```python
from build123d import *

# Parameters (mm, degrees)
F0_R     = 2.5
F1_DEPTH = 4
F2_R     = 2
F3_R     = 1
F4_R     = 0.7
F5_R     = 0.2
F6_R     = 2
F7_R     = 5


with BuildPart() as f1:
    # F0 (on Top) → F1 (new body)
    with BuildSketch(Plane.XY):
        with BuildLine():
            Line((-44, 8.8584928558), (-44, 4.8989794856))
            ThreePointArc((-44, 4.8989794856), (-49.974680765, 0.50254481), (-45, -5))
            Line((-45, -5), (-45, -6.2))
            Line((-45, -6.2), (0, -6.2))
            Line((0, -6.2), (0, -5))
            ThreePointArc((0, -5), (4.974680765, 0.50254481), (-1, 4.8989794856))
            Line((-1, 4.8989794856), (-1, 8.8584928558))
            ThreePointArc((-1, 8.8584928558), (2.3623310777, 10.7048643976), (3.7, 14.3))
            Line((3.7, 14.3), (3.7, 30.6369656558))
            ThreePointArc((3.7, 30.6369656558), (4.7588909504, 35.5339351103), (1.0395584541, 38.8907380037))
            Line((1.0395584541, 38.8907380037), (-4.1791089332, 40))
            Line((-4.1791089332, 40), (-40.8208910668, 40))
            Line((-40.8208910668, 40), (-46.0395584541, 38.8907380037))
            ThreePointArc((-46.0395584541, 38.8907380037), (-49.7588909504, 35.5339351103), (-48.7, 30.6369656558))
            Line((-48.7, 30.6369656558), (-48.7, 14.3))
            ThreePointArc((-48.7, 14.3), (-47.3623310777, 10.7048643976), (-44, 8.8584928558))
        make_face()
        with Locations((-45, 0)):
            Circle(F0_R, mode=Mode.SUBTRACT)
        Circle(F0_R, mode=Mode.SUBTRACT)
        with Locations((-45, 34)):
            Circle(F0_R, mode=Mode.SUBTRACT)
        with Locations((0, 34)):
            Circle(F0_R, mode=Mode.SUBTRACT)
    extrude(amount=F1_DEPTH)

    # F2
    f2_edges = [f1.edges().sort_by_distance(p)[0] for p in [
        (-44, 8.858493, 2),
        (-1, 8.858493, 2),
    ]]
    fillet(f2_edges, radius=F2_R)

    # F3
    f3_edges = [f1.edges().sort_by_distance(p)[0] for p in [
        (-1, 4.898979, 2),
        (-44, 4.898979, 2),
    ]]
    fillet(f3_edges, radius=F3_R)

    # F4
    f4_edges = [f1.edges().sort_by_distance(p)[0] for p in [
        (-45, -5, 2),
        (0, -5, 2),
    ]]
    fillet(f4_edges, radius=F4_R)

    # F5
    f5_edges = [f1.edges().sort_by_distance(p)[0] for p in [
        (-45, -6.2, 2),
        (0, -6.2, 2),
    ]]
    fillet(f5_edges, radius=F5_R)

    # F6
    f6_edges = [f1.edges().sort_by_distance(p)[0] for p in [
        (-48.7, 30.636966, 2),
        (3.7, 30.636966, 2),
    ]]
    fillet(f6_edges, radius=F6_R)

    # F7
    f7_edges = [f1.edges().sort_by_distance(p)[0] for p in [
        (-40.820891, 40, 2),
        (-4.179109, 40, 2),
    ]]
    fillet(f7_edges, radius=F7_R)


solid = f1.part
```
For this review, take the finished solid that the model builds, in its own axes (mm). A direction names the side the tool comes from. Round coordinates to 2 decimals unless told otherwise and drop trailing zeros. Loops run counter-clockwise (first coordinate to the right, second up) from the corner with the lowest first, then second, coordinate; pieces in that order, holes last.
Q1. Insertion check: pin 1 Ø2 at (y, z) = (11.5, 3) entering from -X; pin 2 Ø4 at (x, y) = (-45, 34) entering from +Z; pin 3 Ø1.2 at (y, z) = (22.5, 2.5) entering from +X; pin 4 Ø1.1 at (y, z) = (6.5, 2.5) entering from -X. Each pin has a flat end and moves straight along its axis. Give the tip position at first contact, or say it passes through.
Result sheet:
pin 1: stops at x = -48.4
pin 2: passes through
pin 3: stops at x = 3.7
pin 4: stops at x = -44
Q2. Add section B-B on z = 0.8. Give the number of separate pieces and of enclosed holes in the cut face, plus the area to 3 significant figures.
Result sheet:
separate pieces: 1
enclosed holes: 4
area: 2,290 mm2
Q3. Machinability: for faces 1 (the face through (-47.783, 11.259, 1.972)), 2 (the face through (2.73, 11.18, 1.97)), 3 (the face through (-23, 17, 0)), which of the approach directions +Z, -Z, +X, -X, +Y, -Y give a long, thin tool a straight path to every point of the face, cutting with its end or side? Answer none if there is none.
Result sheet:
face 1: +Z, -Z, -X
face 2: +Z, -Z, +X
face 3: -Z, +X, -X, +Y, -Y
Q4. Mouldability with a two-part tool opening along X and no side actions: class faces 4 (the face through (-23, -6.2, 2)), 5 (the face through (-1.28, 39.384, 1.972)), 6 (the face through (-42.69, -0.96, 1.97)) as +X half, -X half, draft (parallel to the pull), parting line (faces both ways), or undercut.
Result sheet:
face 4: draft
face 5: +X half
face 6: undercut
Q5. Add section D-D on y = 10. Write out the cut boundary in (x, z).
Result sheet:
outline: (-46.63, 0) - (1.63, 0) - (1.63, 4) - (-46.63, 4) - close
Q6. To check wall thickness, follow line 1 along X through (y, z) = (16, 3.4); line 2 along Y through (x, z) = (-47, 1.6); line 3 along X through (y, z) = (7, 1.1). State the ranges of each line that lie inside material, in increasing order.
Result sheet:
line 1: x = -48.7 to 3.7
line 2: y = -4.58 to -1.5, 1.5 to 4.58, 10.32 to 32.5, 35.5 to 38.58
line 3: x = -44 to -1
Q7. Add section C-C on y = 16. Write out the cut boundary in (x, z), plus the area to 3 significant figures.
Result sheet:
outline: (-48.7, 0) - (3.7, 0) - (3.7, 4) - (-48.7, 4) - close
area: 210 mm2
Q8. Add section A-A on y = 0. Write out the cut boundary in (x, z).
Result sheet:
outline: (-50, 0) - (-47.5, 0) - (-47.5, 4) - (-50, 4) - close; (-42.5, 0) - (-2.5, 0) - (-2.5, 4) - (-42.5, 4) - close; (2.5, 0) - (5, 0) - (5, 4) - (2.5, 4) - close
